Input: part model. Units: mm. Frame: model coordinates. Face numbers are marked on the shaded views. A direction names the side the tool comes from. Round coordinates to 2 decimals unless told otherwise and drop trailing zeros. Write each loop counter-clockwise with the first axis right and the second up, starting at its lowest first coordinate (ties: lowest second). Pieces come first, ordered by that corner, then holes. Notation, with made-up numbers: (-4, -38) - (22, -38) arc R22 cw to (22, -27) - close; hole circle Ø7 at (55.5, 1). An arc over 180 degrees is marked (long way). Use one line per item in the form item = value.
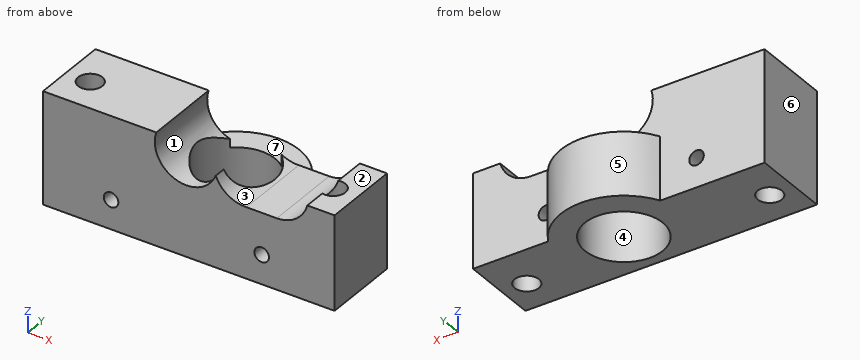
```python
from build123d import *

# Parameters (mm, degrees)
F0_R     = 2.5
F0_R_2   = 8
F1_DEPTH = 23
F2_R     = 1.5
F3_DEPTH = 23.001
F4_W     = 8
F4_H     = 10
F5_DEPTH = 60.001


with BuildPart() as f1:
    # F0 (on Top) → F1 (new body)
    with BuildSketch(Plane.XY):
        with BuildLine():
            Line((-11.5325625947, 6), (-33, 6))
            Line((-33, 6), (-33, -10))
            Line((-33, -10), (27, -10))
            Line((27, -10), (27, 6))
            Line((27, 6), (11.5325625947, 6))
            ThreePointArc((11.5325625947, 6), (0, 13), (-11.5325625947, 6))
        make_face()
        with Locations((-28, -3)):
            Circle(F0_R, mode=Mode.SUBTRACT)
        Circle(F0_R_2, mode=Mode.SUBTRACT)
        with Locations((22, -3)):
            Circle(F0_R, mode=Mode.SUBTRACT)
    extrude(amount=F1_DEPTH)

    # F2 (on face) → F3 (cut, through all)
    with BuildSketch(Plane.XZ.offset(10)):
        with Locations((-19, 6)):
            Circle(F2_R)
        with Locations((12, 6)):
            Circle(F2_R)
        with BuildLine():
            ThreePointArc((2.555311013, 18.6371185947), (2.8878604237, 19.7978189788), (3, 21))
            ThreePointArc((3, 21), (2.8878604237, 22.2021810212), (2.555311013, 23.3628814053))
            ThreePointArc((2.555311013, 23.3628814053), (2.110622026, 21), (2.555311013, 18.6371185947))
        make_face()
        with BuildLine():
            ThreePointArc((2.555311013, 23.3628814053), (2.8878604237, 22.2021810212), (3, 21))
            ThreePointArc((3, 21), (2.8878604237, 19.7978189788), (2.555311013, 18.6371185947))
            ThreePointArc((2.555311013, 18.6371185947), (5.0491141915, 15.5625684423), (8.8639976231, 14.5049402769))
            ThreePointArc((8.8639976231, 14.5049402769), (10.4150204043, 14.7554706749), (11.860622026, 15.3708348754))
            ThreePointArc((11.860622026, 15.3708348754), (8.610622026, 21), (11.860622026, 26.6291651246))
            ThreePointArc((11.860622026, 26.6291651246), (6.4578111185, 27.1331399133), (2.555311013, 23.3628814053))
        make_face()
        with BuildLine():
            ThreePointArc((2.555311013, 18.6371185947), (2.110622026, 21), (2.555311013, 23.3628814053))
            ThreePointArc((2.555311013, 23.3628814053), (-10, 21), (2.555311013, 18.6371185947))
        make_face()
        with BuildLine():
            ThreePointArc((21.2952804645, 23), (17.4442382997, 27.0666494119), (11.860622026, 26.6291651246))
            ThreePointArc((11.860622026, 26.6291651246), (14.2397871506, 24.25), (15.110622026, 21))
            ThreePointArc((15.110622026, 21), (14.2397871506, 17.75), (11.860622026, 15.3708348754))
            ThreePointArc((11.860622026, 15.3708348754), (13.4258145924, 14.7221481451), (15.1054792462, 14.5000020345))
            ThreePointArc((15.1054792462, 14.5000020345), (19.0827263462, 15.854867614), (21.4002303392, 19.3596258759))
            ThreePointArc((21.4002303392, 19.3596258759), (21.5578095538, 20.173094333), (21.610622026, 21))
            ThreePointArc((21.610622026, 21), (21.5313026695, 22.0123537302), (21.2952804645, 23))
        make_face()
        with BuildLine():
            ThreePointArc((15.110622026, 21), (14.2397871506, 24.25), (11.860622026, 26.6291651246))
            ThreePointArc((11.860622026, 26.6291651246), (8.610622026, 21), (11.860622026, 15.3708348754))
            ThreePointArc((11.860622026, 15.3708348754), (14.2397871506, 17.75), (15.110622026, 21))
        make_face()
        with BuildLine():
            ThreePointArc((11.860622026, 15.3708348754), (10.4150204043, 14.7554706749), (8.8639976231, 14.5049402769))
            Line((8.8639976231, 14.5049402769), (15.1054792462, 14.5000020345))
            ThreePointArc((15.1054792462, 14.5000020345), (13.4258145924, 14.7221481451), (11.860622026, 15.3708348754))
        make_face()
        with BuildLine():
            Line((27, 23), (21.2952804645, 23))
            ThreePointArc((21.2952804645, 23), (21.5313026695, 22.0123537302), (21.610622026, 21))
            ThreePointArc((21.610622026, 21), (21.5578095538, 20.173094333), (21.4002303392, 19.3596258759))
            Line((21.4002303392, 19.3596258759), (27, 19.3596258759))
            Line((27, 19.3596258759), (27, 23))
        make_face()
    extrude(amount=-F3_DEPTH, mode=Mode.SUBTRACT)

    # F4 (on face) → F5 (cut, through all)
    with BuildSketch(Plane(origin=(-33, 0, 0), x_dir=(0, -1, 0), z_dir=(-1, 0, 0))):
        with Locations((-10, 18)):
            Rectangle(F4_W, F4_H)
    extrude(amount=-F5_DEPTH, mode=Mode.SUBTRACT)


solid = f1.part
```
(1) Cut plane C-C on z = 17.25. Output: boundary loops of the cut face in (x, y), then the cut area to 3 significant figures.
Derived:
outline = (-33, -10) - (-8.81, -10) - (-8.81, 6) - (-33, 6) - close; (1.81, -10) - (3.3, -10) - (3.3, -7.29) arc R8 cw to (1.81, -7.79) - close; (20.42, -10) - (27, -10) - (27, 6) - (20.42, 6) - (20.42, -1.06) arc R2.5 cw (long way) to (20.42, -4.94) - close; hole circle Ø5 at (-28, -3)
area = 459 mm^2
(2) Material intervals for L1, parallel to Y at x = 22, z = 9.5; L2, parallel to Z at x = 0, y = 10.75; L3, parallel to Z at x = 24, y = 1, sorted ascending.
Derived:
L1 = -10 to -5.5, -0.5 to 6
L2 = 0 to 13
L3 = 0 to 19.36
(3) Draft query along X for the marked faces 4, 5, 6 and 7. Return one class per face: released by +X, released by -X, zero draft, split by the parting line, or undercut.
Derived:
face_4 = undercut
face_5 = split by the parting line
face_6 = released by -X
face_7 = zero draft
(4) Cut plane B-B on y = -3. Output: boundary loops of the cut face in (x, z), then the cut area to 3 significant figures.
Derived:
outline = (-33, 0) - (-30.5, 0) - (-30.5, 23) - (-33, 23) - close; (-25.5, 0) - (-7.42, 0) - (-7.42, 15.81) arc R6.5 cw to (-9.68, 23) - (-25.5, 23) - close; (7.42, 0) - (19.5, 0) - (19.5, 16.21) arc R6.5 cw to (15.11, 14.5) - (8.86, 14.5) arc R6.5 cw to (7.42, 14.61) - close; (24.5, 0) - (27, 0) - (27, 19.36) - (24.5, 19.36) - close; hole circle Ø3 at (-19, 6); hole circle Ø3 at (12, 6)
area = 671 mm^2
(5) Access query for the marked faces 1, 2 and 3. Directions: +Z, -Z, +X, -X, +Y, -Y. A direction counts if a zero-diameter tool reaches every point of the face in a straight line with its end or side. Return the directions, or none.
Derived:
face_1 = +Y, -Y
face_2 = +Z, +X, +Y, -Y
face_3 = +Z, +Y, -Y
(6) Cut plane D-D on y = 1.5. Output: boundary loops of the cut face in (x, z), then the cut area to 3 significant figures.
Derived:
outline = (-33, 0) - (-7.86, 0) - (-7.86, 16.18) arc R6.5 cw to (-9.68, 23) - (-33, 23) - close; (7.86, 0) - (27, 0) - (27, 19.36) - (21.4, 19.36) arc R6.5 cw to (15.11, 14.5) - (8.86, 14.5) arc R6.5 cw to (7.86, 14.54) - close; hole circle Ø3 at (-19, 6); hole circle Ø3 at (12, 6)
area = 866 mm^2
(7) First-contact query: pin 1 Ø6 at (x, z) = (-22.5, 16.5) entering from +Y; pin 2 Ø3 at (x, y) = (-28, -3) entering from -Z; pin 3 Ø3 at (x, y) = (23.5, -3) entering from +Z; pin 4 Ø5.5 at (x, y) = (0, 9) entering from +Z. Flat tips, straight axial feed; report the tip coordinate or a pass-through.
Derived:
pin_1 = 6
pin_2 = through
pin_3 = 19.36
pin_4 = 13
(8) Cut plane A-A on x = -19. Output: boundary loops of the cut face in (y, z), then the cut area to 3 significant figures.
Derived:
outline = (-10, 0) - (6, 0) - (6, 4.5) - (-10, 4.5) - close; (-10, 7.5) - (6, 7.5) - (6, 23) - (-10, 23) - close
area = 320 mm^2
